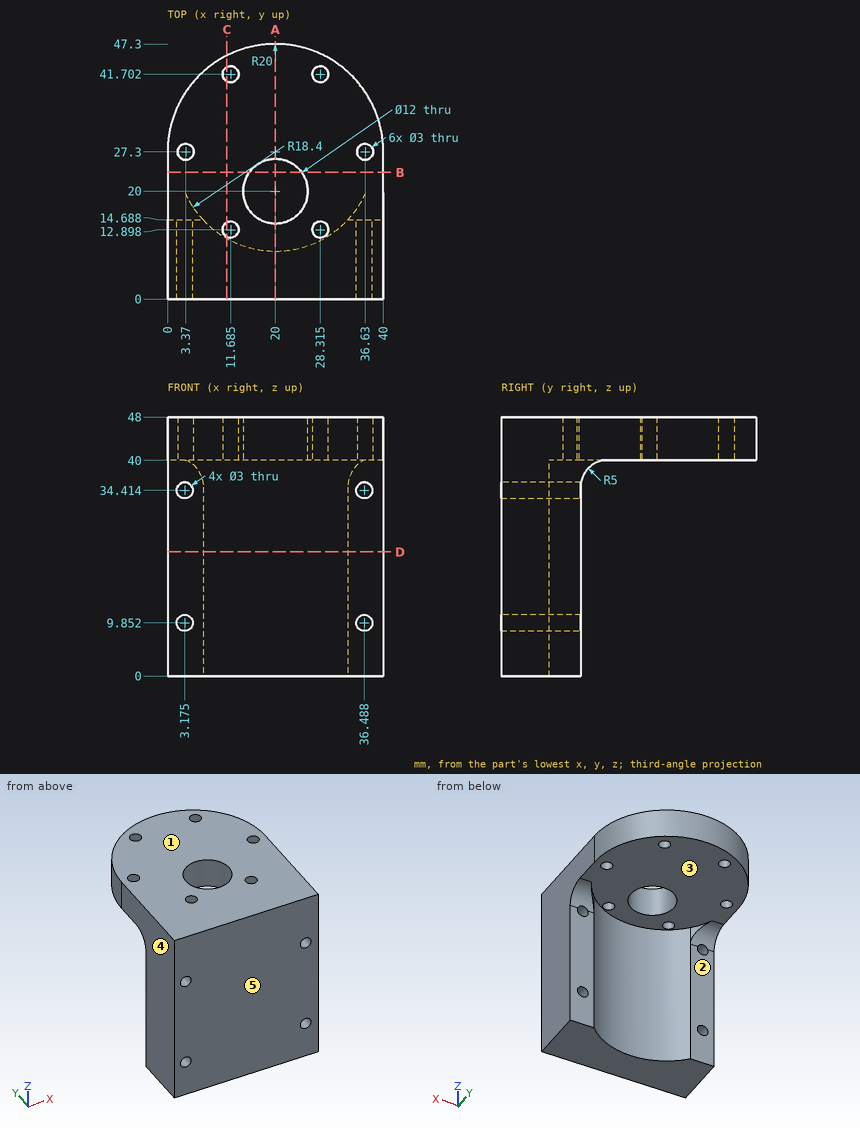
Geometry check sheet. Reference: drawing and pictorial views, mm from the part's lowest x, y, z. A direction names the side the tool comes from. Give positions to 0.01 mm unless a question says otherwise; leave off trailing zeros. Write each loop counter-clockwise with the first axis right and the second up, starting at its lowest first coordinate (ties: lowest second). Pieces come first, ordered by that corner, then holes. Notation, with made-up numbers: M 88.25,-25 L 102.25,-25 A13 ccw 102.25,-13 Z; hole C 65,47.25 d3. An arc over 180 degrees is marked long. Put each result on its own line as item: value. Start each with the question number.
1. Draft check along X on the marked faces 3, 4 and 5. Enter one of: +X half, -X half, draft (parallel to the pull), parting line (faces both ways), or undercut.
2. Section check D-D (z = 23). Record the cut outline in (x, y).
3. Section check C-C (x = 11). Record the cut outline in (y, z).
4. Set-up check for the marked faces 1 and 2: record each of +Z, -Z, +X, -X, +Y, -Y from which the full face is reachable in a straight line by a thin tool's end or side.
5. Go/stop test with flat-tipped pins: pin 1 Ø4 at (x, z) = (36.49, 9.85) entering from +Y; pin 2 Ø10 at (x, z) = (18, 31.5) entering from +Y; pin 3 Ø6 at (x, y) = (4, 42.5) entering from -Z. Record where each tip stops, or that it passes through.
6. Section check B-B (y = 23.5). Record the cut outline in (x, z).
7. Section check A-A (x = 20). Record the cut outline in (y, z).
8. Scan lines: line 1 along Z through (x, y) = (29.5, 19.5); line 2 along Y through (x, z) = (20, 42.5); line 3 along Y through (x, z) = (37, 26). Record each from-to range of solid material in increasing order. Write a range as [from, to].
Answer list:
1. face 3: undercut
1. face 4: -X half
1. face 5: draft
2. outline: M 0,0 L 40,0 L 40,14.69 L 33.4,14.69 A18.4 cw 6.6,14.69 L 0,14.69 Z
3. outline: M 0,0 L 11.25,0 L 11.25,40 L 11.56,40 L 11.56,48 L 0,48 Z; M 14.23,40 L 40.37,40 L 40.37,48 L 14.23,48 Z; M 43.04,40 L 45.16,40 L 45.16,48 L 43.04,48 Z
4. face 1: +Z, +X, -X, +Y, -Y
4. face 2: -Z, +X, -X, +Y
5. pin 1: y = 14.69
5. pin 2: y = 10.28
5. pin 3: z = 40
6. outline: M 0,40 L 15.13,40 L 15.13,48 L 0,48 Z; M 24.87,40 L 40,40 L 40,48 L 24.87,48 Z
7. outline: M 0,0 L 8.9,0 L 8.9,40 L 14,40 L 14,48 L 0,48 Z; M 26,40 L 47.3,40 L 47.3,48 L 26,48 Z
8. line 1: [40, 48]
8. line 2: [0, 14], [26, 47.3]
8. line 3: [0, 14.69]
